Read the model definition and answer for the solid it produces. Units are mm, in the model's axes. Coordinates: 2 decimals unless noted, no trailing zeros. Write each loop counter-clockwise with the first axis right and the second up, starting at its lowest first coordinate (ties: lowest second). Pieces come first, ordered by that corner, then holes.
from build123d import *

# Parameters (mm, degrees)
SKETCH2_R           = 2
BOSS_EXTRUDE1_DEPTH = 1


with BuildPart() as part:
    # Sketch2 → Boss-Extrude1 (new body)
    with BuildSketch(Plane(origin=(0, 0, 0), x_dir=(1, 0, 0), z_dir=(0, 1, 0))):
        with BuildLine():
            ThreePointArc((-22.173324826, 6.110946422), (-16.263455967, -16.263455967), (6.110946422, -22.173324826))
            Line((6.110946422, -22.173324826), (22.173324826, -6.110946422))
            ThreePointArc((22.173324826, -6.110946422), (16.263455967, 16.263455967), (-6.110946422, 22.173324826))
            Line((-6.110946422, 22.173324826), (-22.173324826, 6.110946422))
        make_face()
        with BuildLine():
            ThreePointArc((0, 15), (10.606601718, 10.606601718), (15, 0))
            ThreePointArc((15, 0), (10.606601718, -10.606601718), (0, -15))
            ThreePointArc((0, -15), (-10.606601718, -10.606601718), (-15, 0))
            ThreePointArc((-15, 0), (-10.606601718, 10.606601718), (0, 15))
        make_face(mode=Mode.SUBTRACT)
        with Locations((-19, 0)):
            Circle(SKETCH2_R, mode=Mode.SUBTRACT)
        with Locations((0, 19)):
            Circle(SKETCH2_R, mode=Mode.SUBTRACT)
        with Locations((0, -19)):
            Circle(SKETCH2_R, mode=Mode.SUBTRACT)
        with Locations((19, 0)):
            Circle(SKETCH2_R, mode=Mode.SUBTRACT)
    extrude(amount=BOSS_EXTRUDE1_DEPTH)


solid = part.part
Item 1: Determine the mould class of faces 1 (the cylindrical face through (16.502, 0.493, -16.022)), 2 (the cylindrical face through (-0.26, 0.493, 17.017)), 3 (the flat face through (-14.03, 0.493, -14.255)) for opening direction X: +X half, -X half, draft (parallel to the pull), parting line (faces both ways), or undercut.
Item 2: The part is cut by section A-A (y = 0.55). Give the vertices of the cut face in (x, z), and give its area (3 significant figures).
Item 3: Find the intervals of material crossed by probe 1 along X at (y, z) = (0.9, -7); probe 2 along X at (y, z) = (0.2, -19); probe 3 along Z at (x, y) = (19, 0.4), in increasing order.
Item 4: The part is cut by section C-C (z = -19). Give the vertices of the cut face in (x, y).
Item 5: The part is cut by section B-B (x = 19). Give the vertices of the cut face in (y, z).
Item 6: Given pin 1 (4 mm diameter, centred on x = -15, z = -18, fed in from -Y), flat-ended and moving along its own axis, determine where the tip first touches the part or whether it passes through.
Answer:
1. face 1: parting line
1. face 2: undercut
1. face 3: -X half
2. outline: (-22.17, -6.11) - (-6.11, -22.17) arc R23 ccw to (22.17, 6.11) - (6.11, 22.17) arc R23 ccw to start; hole circle Ø4 at (-19, 0); hole circle Ø30 at (0, 0); hole circle Ø4 at (0, -19); hole circle Ø4 at (0, 19); hole circle Ø4 at (19, 0)
2. area: 813 mm2
3. probe 1: x = -21.28 to -13.27, 13.27 to 21.91
3. probe 2: x = -9.28 to -2, 2 to 12.96
3. probe 3: z = -12.96 to -2, 2 to 9.28
4. outline: (-9.28, 0) - (-2, 0) - (-2, 1) - (-9.28, 1) - close; (2, 0) - (12.96, 0) - (12.96, 1) - (2, 1) - close
5. outline: (0, -12.96) - (1, -12.96) - (1, -2) - (0, -2) - close; (0, 2) - (1, 2) - (1, 9.28) - (0, 9.28) - close
6. pin 1: passes through
